Verification items for the finished model (mm, model axes). A direction names the side the tool comes from. Coordinates: 2 decimals unless noted, no trailing zeros. Write each loop counter-clockwise with the first axis right and the second up, starting at its lowest first coordinate (ties: lowest second). Pieces come first, ordered by that corner, then holes. Notation, with made-up numbers: M 27,-40 L 64,-40 A24 cw 64,-19 Z; hole C 20,-19 d3. An arc over 180 degrees is marked long. Answer in a Markdown table with one row per item.
from build123d import *
from build123d.topology import SkipClean

# Parameters (mm, degrees)
SKETCH1_R               = 1.5
BOSS_EXTRUDE1_DEPTH     = 2.2
SKETCH3_R               = 4.3
SKETCH3_R_2             = 2.7
BOSS_EXTRUDE2_DEPTH     = 5.6
BOSS_EXTRUDE3_START     = 0.2
SKETCH4_R               = 6.4
SKETCH4_R_2             = 2.7
BOSS_EXTRUDE3_DEPTH     = 0.2
SKETCH7_R               = 2.7
CUT_EXTRUDE1_DEPTH      = 1.5
CUT_EXTRUDE2_REACH      = 31.527
SKETCH8_R               = 0.75
LPATTERN1_COUNT         = 5
LPATTERN1_PITCH         = 3.5
MIRROR1_COPY_1_REACH    = 31.527
MIRROR1_COPY_1_SKETCH_R = 0.75
MIRROR1_COPY_2_REACH    = 31.527
MIRROR1_COPY_2_SKETCH_R = 0.75
MIRROR1_COPY_3_REACH    = 31.527
MIRROR1_COPY_3_SKETCH_R = 0.75
MIRROR1_COPY_4_REACH    = 31.527
MIRROR1_COPY_4_SKETCH_R = 0.75


with BuildPart() as part:
    # Sketch1 → Boss-Extrude1 (new body)
    with BuildSketch(Plane(origin=(0, 0, 0), x_dir=(1, 0, 0), z_dir=(0, 1, 0))):
        with BuildLine():
            Line((-1.473634962, 26.53), (-6.287509169, 1.194666667))
            ThreePointArc((-6.287509169, 1.194666667), (-6.4, 0), (-6.287509169, -1.194666667))
            Line((-6.287509169, -1.194666667), (-1.473634962, -26.53))
            ThreePointArc((-1.473634962, -26.53), (0, -27.75), (1.473634962, -26.53))
            Line((1.473634962, -26.53), (6.287509169, -1.194666667))
            ThreePointArc((6.287509169, -1.194666667), (6.4, 0), (6.287509169, 1.194666667))
            Line((6.287509169, 1.194666667), (1.473634962, 26.53))
            ThreePointArc((1.473634962, 26.53), (0, 27.75), (-1.473634962, 26.53))
        make_face()
        with Locations(Location((0, 0, 0), (0, 0, 270))):
            Circle(SKETCH1_R, mode=Mode.SUBTRACT)
    extrude(amount=BOSS_EXTRUDE1_DEPTH)

    # Sketch3 → Boss-Extrude2 (add)
    with BuildSketch(Plane(origin=(0, 2.2, 0), x_dir=(1, 0, 0), z_dir=(0, 1, 0))):
        with Locations(Location((0, 0, 0), (0, 0, 270))):
            Circle(SKETCH3_R)
        with Locations(Location((0, 0, 0), (0, 0, 270))):
            Circle(SKETCH3_R_2, mode=Mode.SUBTRACT)
    extrude(amount=BOSS_EXTRUDE2_DEPTH)

    # Sketch4 → Boss-Extrude3 (add)
    with SkipClean():  # the faces are left unmerged after this step: merging them gives an invalid solid
        with BuildSketch(Plane.XZ.offset(BOSS_EXTRUDE3_START)):
            with Locations(Location((0, 0, 0), (0, 0, 270))):
                Circle(SKETCH4_R)
            with Locations(Location((0, 0, 0), (0, 0, 90))):
                Circle(SKETCH4_R_2, mode=Mode.SUBTRACT)
        extrude(amount=-BOSS_EXTRUDE3_DEPTH)

    # Sketch7 → Cut-Extrude1 (cut)
    with SkipClean():  # the faces are left unmerged after this step: merging them gives an invalid solid
        with BuildSketch(Plane.XZ):
            with Locations(Location((0, 0, 0), (0, 0, 90))):
                Circle(SKETCH7_R)
        extrude(amount=-CUT_EXTRUDE1_DEPTH, mode=Mode.SUBTRACT)

    # Sketch8 → Cut-Extrude2 (cut, up to next)
    with BuildSketch(Plane.XZ, mode=Mode.PRIVATE) as cut_extrude2_sk1:
        with Locations(Location((0, 12.25, 0), (0, 0, 270))):
            Circle(SKETCH8_R)
    cut_extrude2_tool1 = extrude(cut_extrude2_sk1.sketch, amount=-CUT_EXTRUDE2_REACH, mode=Mode.PRIVATE) & part.part
    cut_extrude2 = cut_extrude2_tool1.solids().sort_by_distance((0, 0, 12.25))[0]
    add(cut_extrude2, mode=Mode.SUBTRACT)

    # LPattern1: Cut-Extrude2 ×5
    with SkipClean():  # the faces are left unmerged after this step: merging them gives an invalid solid
        with Locations(*[(0, 0, i * LPATTERN1_PITCH) for i in range(1, LPATTERN1_COUNT)]):
            add(cut_extrude2, mode=Mode.SUBTRACT)

    # Mirror1: Cut-Extrude2 across plane
    with SkipClean():  # the faces are left unmerged after this step: merging them gives an invalid solid
        add(cut_extrude2.mirror(Plane.XY), mode=Mode.SUBTRACT)

    # Mirror1 copy 1 sketch → Mirror1 copy 1 (cut, up to next)
    with BuildSketch(Plane(origin=(0, 0, -3.5), x_dir=(1, 0, 0), z_dir=(0, -1, 0)), mode=Mode.PRIVATE) as mirror1_copy_1_sk1:
        with Locations((0, -12.25)):
            Circle(MIRROR1_COPY_1_SKETCH_R)
    mirror1_copy_1_tool1 = extrude(mirror1_copy_1_sk1.sketch, amount=-MIRROR1_COPY_1_REACH, mode=Mode.PRIVATE) & part.part
    add(mirror1_copy_1_tool1.solids().sort_by_distance((0, 0, -15.75))[0], mode=Mode.SUBTRACT)

    # Mirror1 copy 2 sketch → Mirror1 copy 2 (cut, up to next)
    with BuildSketch(Plane(origin=(0, 0, -7), x_dir=(1, 0, 0), z_dir=(0, -1, 0)), mode=Mode.PRIVATE) as mirror1_copy_2_sk1:
        with Locations((0, -12.25)):
            Circle(MIRROR1_COPY_2_SKETCH_R)
    mirror1_copy_2_tool1 = extrude(mirror1_copy_2_sk1.sketch, amount=-MIRROR1_COPY_2_REACH, mode=Mode.PRIVATE) & part.part
    add(mirror1_copy_2_tool1.solids().sort_by_distance((0, 0, -19.25))[0], mode=Mode.SUBTRACT)

    # Mirror1 copy 3 sketch → Mirror1 copy 3 (cut, up to next)
    with BuildSketch(Plane(origin=(0, 0, -10.5), x_dir=(1, 0, 0), z_dir=(0, -1, 0)), mode=Mode.PRIVATE) as mirror1_copy_3_sk1:
        with Locations((0, -12.25)):
            Circle(MIRROR1_COPY_3_SKETCH_R)
    mirror1_copy_3_tool1 = extrude(mirror1_copy_3_sk1.sketch, amount=-MIRROR1_COPY_3_REACH, mode=Mode.PRIVATE) & part.part
    add(mirror1_copy_3_tool1.solids().sort_by_distance((0, 0, -22.75))[0], mode=Mode.SUBTRACT)

    # Mirror1 copy 4 sketch → Mirror1 copy 4 (cut, up to next)
    with BuildSketch(Plane(origin=(0, 0, -14), x_dir=(1, 0, 0), z_dir=(0, -1, 0)), mode=Mode.PRIVATE) as mirror1_copy_4_sk1:
        with Locations((0, -12.25)):
            Circle(MIRROR1_COPY_4_SKETCH_R)
    mirror1_copy_4_tool1 = extrude(mirror1_copy_4_sk1.sketch, amount=-MIRROR1_COPY_4_REACH, mode=Mode.PRIVATE) & part.part
    add(mirror1_copy_4_tool1.solids().sort_by_distance((0, 0, -26.25))[0], mode=Mode.SUBTRACT)


solid = part.part
1) Sectioned sample at A-A (z = 0). Record the cut outline in (x, y).
Response values:
| item | result |
|---|---|
| outline | M -6.4,-0.2 L -2.7,-0.2 L -2.7,1.5 L -1.5,1.5 L -1.5,2.2 L -2.7,2.2 L -2.7,7.8 L -4.3,7.8 L -4.3,2.2 L -6.4,2.2 Z; M 1.5,1.5 L 2.7,1.5 L 2.7,-0.2 L 6.4,-0.2 L 6.4,2.2 L 4.3,2.2 L 4.3,7.8 L 2.7,7.8 L 2.7,2.2 L 1.5,2.2 Z |
2) Tool access check on faces 1 (the face through (1.2, 2.2, 1.2)), 2 (the face through (-3.914, 1.085, 13.685)), 3 (the face through (1.2, 1.5, 1.2)). Record the directions out of +Z, -Z, +X, -X, +Y, -Y that give a thin tool (end or side, any length) a straight path to the whole face; none if there is none.
Response values:
| item | result |
|---|---|
| face 1 | +Y |
| face 2 | +Z, -X, +Y, -Y |
| face 3 | -Y |
3) Release check for a two-part mould opening along X. For faces 4 (the face through (3.847, 1.085, 14.04)), 5 (the face through (-0.163, 1.085, -23.482)), 6 (the face through (-3.847, 1.085, -14.04)) record: +X half, -X half, draft (parallel to the pull), parting line (faces both ways), or undercut.
Response values:
| item | result |
|---|---|
| face 4 | +X half |
| face 5 | undercut |
| face 6 | -X half |
4) Depth check by flat-ended pin: pin 1 (2 mm diameter, centred on x = -3, z = 10, fed in from -Y); pin 2 (2 mm diameter, centred on x = 0, z = -15.75, fed in from +Y); pin 3 (6 mm diameter, centred on x = -1, z = -1, fed in from -Y); pin 4 (3.5 mm diameter, centred on x = 0, z = 0, fed in from -Y). Enter the tip coordinate at first touch or a pass-through.
Response values:
| item | result |
|---|---|
| pin 1 | stops at y = 0 |
| pin 2 | stops at y = 2.2 |
| pin 3 | stops at y = -0.2 |
| pin 4 | stops at y = 1.5 |
5) Sectioned sample at B-B (y = 1). Give the number of separate pieces and of enclosed holes in the cut face, then the cut area to 3 significant figures.
Response values:
| item | result |
|---|---|
| separate pieces | 1 |
| enclosed holes | 11 |
| area | 388 mm² |
6) Sectioned sample at D-D (y = 5.25). Record the cut outline in (x, z).
Response values:
| item | result |
|---|---|
| outline | C 0,0 d8.6; hole C 0,0 d5.4 |
7) Thickness scan on L1, parallel to Z at x = 0.25, y = 4.75; L2, parallel to Y at x = -4.75, z = 3.5; L3, parallel to Y at x = 1.75, z = 15. Record the ranges inside material, lowest first. Write a range as [from, to].
Response values:
| item | result |
|---|---|
| L1 | z = [-4.29, -2.69], [2.69, 4.29] |
| L2 | y = [-0.2, 2.2] |
| L3 | y = [0, 2.2] |
